Build history of the part. All positions in model axes, mm. Face numbers are marked on the shaded views. A direction names the side the tool comes from. Coordinates: 2 decimals unless noted, no trailing zeros. Loops run counter-clockwise (first coordinate to the right, second up) from the corner with the lowest first, then second, coordinate; pieces in that order, holes last.
Item 1: Drill centre lines: line 1 along Z through (x, y) = (37, 7); line 2 along Y through (x, z) = (-40.5, -40); line 3 along Y through (x, z) = (-29.5, 16). Where is each one in solid material? Low to high.
Item 2: Mould opens along X. For the marked faces 1, 2 and 3 say: released by +X, released by -X, zero draft, split by the parting line, or undercut.
Item 3: Cut at D-D (x = -27). List the corners of the cut face in (y, z), and give its area (3 significant figures).
Item 4: Cut at C-C (z = -23). List the corners of the cut face in (x, y).
Item 5: Flat gauge pins, fed straight in: pin 1 (2 mm diameter, centred on x = -40, y = -28, fed in from +Z); pin 2 (8 mm diameter, centred on x = 7.5, y = -41.5, fed in from +Z); pin 3 (6 mm diameter, centred on x = -22.5, z = -17, fed in from -Y). Where does each tip first touch, or does it go through?
Item 6: 3-axis set-ups, long thin cutter, end or side, ignore diameter. For the marked faces 4 and 5: which of +Z, -Z, +X, -X, +Y, -Y reach the whole face in a straight line?
Item 7: Cut at A-A (y = -7.5). List the corners of the cut face in (x, z).
Item 8: Cut at B-B (x = 0). List the corners of the cut face in (y, z).
from build123d import *

# Parameters (mm, degrees)
F0_W          = 90
F0_H          = 90
F1_DEPTH      = 30
F1_DEPTH_BACK = 30
F2_R          = 13
F3_DEPTH      = 4
F2_R_2        = 2.5
F4_DEPTH      = 60
F2_R_3        = 6
F5_DEPTH      = 28
F6_R          = 8


with BuildPart() as f1:
    # F0 (on Front) → F1 (new body, two sides)
    with BuildSketch(Plane.XZ) as f1_sk:
        Rectangle(F0_W, F0_H)
    extrude(amount=F1_DEPTH)
    extrude(f1_sk.sketch, amount=-F1_DEPTH_BACK)

    # F2 (on face) → F3 (cut)
    with BuildSketch(Plane.XZ.offset(30)):
        with BuildLine():
            Line((-25.685599, 27.5), (-45, 27.5))
            Line((-45, 27.5), (-45, -27.5))
            Line((-45, -27.5), (-25.685599, -27.5))
            ThreePointArc((-25.685599, -27.5), (0, -42), (25.685599, -27.5))
            Line((25.685599, -27.5), (45, -27.5))
            Line((45, -27.5), (45, 27.5))
            Line((45, 27.5), (25.685599, 27.5))
            ThreePointArc((25.685599, 27.5), (0, 42), (-25.685599, 27.5))
        make_face()
        with Locations((0, 19)):
            Circle(F2_R, mode=Mode.SUBTRACT)
    extrude(amount=-F3_DEPTH, mode=Mode.SUBTRACT)

    # F2 (on face) → F4 (cut)
    with BuildSketch(Plane.XZ.offset(30)):
        with Locations((-37, 37)):
            Circle(F2_R_2)
        with Locations((37, 37)):
            Circle(F2_R_2)
        with Locations((37, -37)):
            Circle(F2_R_2)
        with Locations((-37, -37)):
            Circle(F2_R_2)
    extrude(amount=-F4_DEPTH, mode=Mode.SUBTRACT)

    # F2 (on face) → F5 (join)
    with BuildSketch(Plane.XZ.offset(30)):
        with Locations((0, 19)):
            Circle(F2_R_3)
    extrude(amount=F5_DEPTH)

    # F6
    f6_edges = [f1.edges().sort_by_distance(p)[0] for p in [
        (45, 0, 45),
        (45, 0, -45),
        (-45, 0, -45),
        (-45, 0, 45),
    ]]
    fillet(f6_edges, radius=F6_R)


solid = f1.part
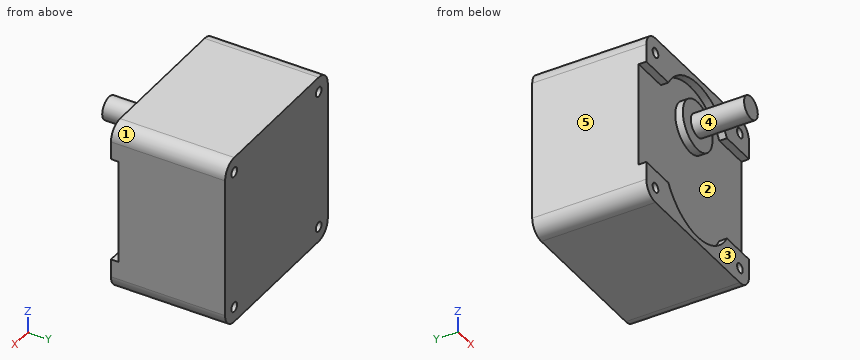
Filled sheet:
1. line 1: z = -45 to -39.5, -34.5 to 34.5, 39.5 to 45
1. line 2: y = -30 to 30
1. line 3: y = -26 to 30
2. face 1: released by +X
2. face 2: undercut
2. face 3: zero draft
3. outline: (-30, -45) - (30, -45) - (30, 45) - (-30, 45) - (-30, 27.5) - (-26, 27.5) - (-26, -27.5) - (-30, -27.5) - close
3. area: 5,180 mm2
4. outline: (-45, -26) - (45, -26) - (45, 30) - (-45, 30) - close
5. pin 1: stops at z = 44.75
5. pin 2: stops at z = 23.87
5. pin 3: stops at y = -26
6. face 4: -Y
6. face 5: +Z, -Z, -X, +Y, -Y
7. outline: (-45, -37) arc R8 ccw to (-37, -45) - (37, -45) arc R8 ccw to (45, -37) - (45, 37) arc R8 ccw to (37, 45) - (-37, 45) arc R8 ccw to (-45, 37) - close; hole circle Ø5 at (-37, -37); hole circle Ø5 at (-37, 37); hole circle Ø5 at (37, -37); hole circle Ø5 at (37, 37)
8. outline: (-58, 13) - (-30, 13) - (-30, 6) - (-26, 6) - (-26, -42) - (-30, -42) - (-30, -45) - (30, -45) - (30, 45) - (-30, 45) - (-30, 42) - (-26, 42) - (-26, 32) - (-30, 32) - (-30, 25) - (-58, 25) - close
